Can you work these out from the model? Positions are in its coordinate system, mm. Face numbers are marked on the shaded views. A direction names the side the tool comes from. Coordinates: 2 decimals unless noted, no trailing zeros. Loops run counter-clockwise (first coordinate to the right, second up) from the corner with the lowest first, then second, coordinate; pieces in that order, holes last.
```python
from build123d import *
from OCP.BRepFilletAPI import BRepFilletAPI_MakeChamfer

# Parameters (mm, degrees)
SKETCH1_W                    = 2.54
SKETCH1_H                    = 2.54
BOSS_EXTRUDE1_DEPTH          = 2.54
BOSS_EXTRUDE2_START          = -5.64
SKETCH2_W                    = 0.65
SKETCH2_H                    = 0.65
BOSS_EXTRUDE2_DEPTH          = 11.34
CHAMFER1_SIZE                = 0.3
CHAMFER1_SIZE2               = 0.091719204
CHAMFER3_SIZE                = 0.7
CHAMFER3_SIZE2               = 0.341412812
CHAMFER4_SIZE                = 0.7
CHAMFER4_SIZE2               = 0.341412812
R_P_TITION_START             = -1.27
R_P_TITION_LIN_AIRE3_DEPTH   = 2.54
R_P_TITION_START_2           = -0.325
R_P_TITION_LIN_AIRE3_2_DEPTH = 0.65
R_P_TITION_START_3           = 1.611412812
R_P_TITION_LIN_AIRE3_3_DEPTH = 4.397174376
R_P_TITION_START_4           = -1
R_P_TITION_LIN_AIRE3_4_DEPTH = 5


with BuildPart() as part:
    # Sketch1 → Boss-Extrude1 (new body)
    with BuildSketch(Plane(origin=(0, 0, 0), x_dir=(1, 0, 0), z_dir=(0, 1, 0))):
        Rectangle(SKETCH1_W, SKETCH1_H)
    extrude(amount=BOSS_EXTRUDE1_DEPTH)

    # Sketch2 → Boss-Extrude2 (add)
    with BuildSketch(Plane(origin=(0, 2.54, 0), x_dir=(1, 0, 0), z_dir=(0, 1, 0)).offset(BOSS_EXTRUDE2_START)):
        Rectangle(SKETCH2_W, SKETCH2_H)
    extrude(amount=BOSS_EXTRUDE2_DEPTH)

    # Chamfer1: one chamfer whose edges measure the first distance from different faces: ONE call of the kernel's chamfer builder (chamfer() names one face for all edges)
    chamfer1_edges_1 = [part.edges().sort_by_distance(p)[0] for p in [
        (-0.325, -3.1, 0),
        (0, -3.1, -0.325),
        (0.325, -3.1, 0),
        (0, -3.1, 0.325),
    ]]
    chamfer1_side_1 = [part.faces().sort_by_distance(p)[0] for p in [
        (0, -3.1, 0),
    ]]
    chamfer1_edges_2 = [part.edges().sort_by_distance(p)[0] for p in [
        (-0.325, 8.24, 0),
    ]]
    chamfer1_side_2 = [part.faces().sort_by_distance(p)[0] for p in [
        (-0.325, 5.39, 0),
    ]]
    chamfer1_edges_3 = [part.edges().sort_by_distance(p)[0] for p in [
        (0, 8.24, 0.325),
    ]]
    chamfer1_side_3 = [part.faces().sort_by_distance(p)[0] for p in [
        (0, 5.39, 0.325),
    ]]
    chamfer1_edges_4 = [part.edges().sort_by_distance(p)[0] for p in [
        (0.325, 8.24, 0),
    ]]
    chamfer1_side_4 = [part.faces().sort_by_distance(p)[0] for p in [
        (0.325, 5.39, 0),
    ]]
    chamfer1_edges_5 = [part.edges().sort_by_distance(p)[0] for p in [
        (0, 8.24, -0.325),
    ]]
    chamfer1_side_5 = [part.faces().sort_by_distance(p)[0] for p in [
        (0, 5.39, -0.325),
    ]]
    chamfer1 = BRepFilletAPI_MakeChamfer(part.part.solid().wrapped)
    for e in chamfer1_edges_1:
        chamfer1.Add(CHAMFER1_SIZE, CHAMFER1_SIZE2, e.wrapped, chamfer1_side_1[0].wrapped)  # the first distance lies on this face
    for e in chamfer1_edges_2:
        chamfer1.Add(CHAMFER1_SIZE, CHAMFER1_SIZE2, e.wrapped, chamfer1_side_2[0].wrapped)  # the first distance lies on this face
    for e in chamfer1_edges_3:
        chamfer1.Add(CHAMFER1_SIZE, CHAMFER1_SIZE2, e.wrapped, chamfer1_side_3[0].wrapped)  # the first distance lies on this face
    for e in chamfer1_edges_4:
        chamfer1.Add(CHAMFER1_SIZE, CHAMFER1_SIZE2, e.wrapped, chamfer1_side_4[0].wrapped)  # the first distance lies on this face
    for e in chamfer1_edges_5:
        chamfer1.Add(CHAMFER1_SIZE, CHAMFER1_SIZE2, e.wrapped, chamfer1_side_5[0].wrapped)  # the first distance lies on this face
    add(Compound.cast(chamfer1.Shape()), mode=Mode.REPLACE)

    # Chamfer3
    chamfer3_edges = [part.edges().sort_by_distance(p)[0] for p in [
        (1.27, 2.54, 0),
        (1.27, 1.27, 1.27),
        (1.27, 1.27, -1.27),
    ]]
    chamfer3_side = [part.faces().sort_by_distance(p)[0] for p in [
        (1.27, 1.27, 0),
    ]]
    chamfer(chamfer3_edges, length=CHAMFER3_SIZE, length2=CHAMFER3_SIZE2, reference=chamfer3_side[0])

    # Chamfer4
    chamfer4_edges = [part.edges().sort_by_distance(p)[0] for p in [
        (-1.27, 2.54, 0),
        (-1.27, 1.27, 1.27),
        (-1.27, 1.27, -1.27),
    ]]
    chamfer4_side = [part.faces().sort_by_distance(p)[0] for p in [
        (-1.27, 1.27, 0),
    ]]
    chamfer(chamfer4_edges, length=CHAMFER4_SIZE, length2=CHAMFER4_SIZE2, reference=chamfer4_side[0])

    # Répétition linéaire3: read off the stored shape, not the designer's step
    # Répétition linéaire3 outline → Répétition linéaire3 (add)
    with BuildSketch(Plane.XY.offset(R_P_TITION_START)):
        Polygon((3.468587188, 2.54), (1.611412812, 2.54), (1.27, 1.84), (1.27, 0), (6.35, 0), (6.35, 1.84), (6.008587188, 2.54), (4.151412812, 2.54), (3.81, 1.84), align=None)
    extrude(amount=R_P_TITION_LIN_AIRE3_DEPTH)

    # R_p_tition lin_aire3 2 outline → R_p_tition lin_aire3 2 (add)
    with BuildSketch(Plane.XY.offset(R_P_TITION_START_2)):
        Polygon((2.215, 7.94), (2.215, 2.54), (2.865, 2.54), (2.865, 7.94), (2.773280796, 8.24), (2.306719204, 8.24), align=None)
        Polygon((2.865, 0), (2.215, 0), (2.215, -3.008280796), (2.515, -3.1), (2.565, -3.1), (2.865, -3.008280796), align=None)
        Polygon((5.405, 0), (4.755, 0), (4.755, -3.008280796), (5.055, -3.1), (5.105, -3.1), (5.405, -3.008280796), align=None)
        Polygon((4.755, 7.94), (4.755, 2.54), (5.405, 2.54), (5.405, 7.94), (5.313280796, 8.24), (4.846719204, 8.24), align=None)
    extrude(amount=R_P_TITION_LIN_AIRE3_2_DEPTH)

    # R_p_tition lin_aire3 3 outline → R_p_tition lin_aire3 3 (cut)
    with BuildSketch(Plane.YZ.offset(R_P_TITION_START_3)):
        Polygon((-3.1, 0.025), (-3.008280796, 0.325), (-3.1, 0.325), align=None)
        Polygon((-3.008280796, -0.325), (-3.1, -0.025), (-3.1, -0.325), align=None)
        Polygon((8.24, 0.325), (7.94, 0.325), (8.24, 0.233280796), align=None)
        Polygon((8.24, -0.325), (8.24, -0.233280796), (7.94, -0.325), align=None)
    extrude(amount=R_P_TITION_LIN_AIRE3_3_DEPTH, mode=Mode.SUBTRACT)

    # R_p_tition lin_aire3 4 outline → R_p_tition lin_aire3 4 (cut)
    with BuildSketch(Plane(origin=(0, 0, 0), x_dir=(1, 0, 0), z_dir=(0, 1, 0)).offset(R_P_TITION_START_4)):
        Polygon((4.151412812, -1.27), (3.81, -0.57), (3.468587188, -1.27), align=None)
        Polygon((1.27, 0.57), (1.611412812, 1.27), (1.27, 1.27), align=None)
        Polygon((3.81, 0.57), (4.151412812, 1.27), (3.468587188, 1.27), align=None)
        Polygon((6.008587188, 1.27), (6.35, 0.57), (6.35, 1.27), align=None)
        Polygon((6.35, -0.57), (6.008587188, -1.27), (6.35, -1.27), align=None)
        Polygon((1.27, -1.27), (1.611412812, -1.27), (1.27, -0.57), align=None)
    extrude(amount=R_P_TITION_LIN_AIRE3_4_DEPTH, mode=Mode.SUBTRACT)


solid = part.part
```
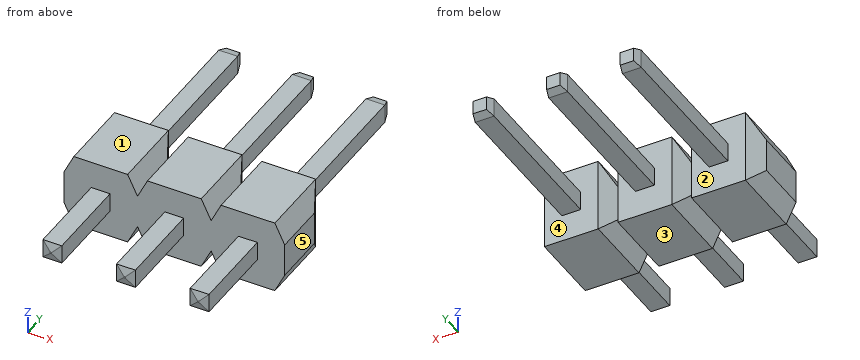
(1) If we mould it in two halves opening along X, with no side actions, what happens to the marked faces 3, 4 and 5? For each: released by +X, released by -X, zero draft, split by the parting line, or undercut.
Check values:
face 3: zero draft
face 4: undercut
face 5: released by +X
(2) Which directions (+Z, -Z, +X, -X, +Y, -Y) give clear straight access to the entire face, cutting with the end or side of a thin tool? Please do the marked faces 1 and 2.
Check values:
face 1: +Z, +X, -X, +Y, -Y
face 2: +Y
(3) I'm going to push flat-ended pins straight in: pin 1 (1.5 mm diameter, centred on y = 5.5, z = -1, fed in from -X) (3 decimals); pin 2 (0.5 mm diameter, centred on x = 2.5, y = 4, fed in from -Z) (3 decimals); pin 3 (0.5 mm diameter, centred on x = 2.5, y = 5, fed in from +Z) (3 decimals). Where does each tip first touch, or does it pass through?
Check values:
pin 1: stops at x = -0.325
pin 2: stops at z = -0.325
pin 3: stops at z = 0.325
(4) I want a section at B-B on z = -0.8. Write out the boundary of the cut face in (x, y).
Check values:
outline: (-1.16, 0) - (1.16, 0) - (1.16, 2.07) - (0.93, 2.54) - (-0.93, 2.54) - (-1.16, 2.07) - close; (1.38, 0) - (3.7, 0) - (3.7, 2.07) - (3.47, 2.54) - (1.61, 2.54) - (1.38, 2.07) - close; (3.92, 0) - (6.24, 0) - (6.24, 2.07) - (6.01, 2.54) - (4.15, 2.54) - (3.92, 2.07) - close
(5) I want a section at A-A on y = 0.75. Write out the boundary of the cut face in (x, z).
Check values:
outline: (-1.27, -0.57) - (-0.93, -1.27) - (0.93, -1.27) - (1.27, -0.57) - (1.61, -1.27) - (3.47, -1.27) - (3.81, -0.57) - (4.15, -1.27) - (6.01, -1.27) - (6.35, -0.57) - (6.35, 0.57) - (6.01, 1.27) - (4.15, 1.27) - (3.81, 0.57) - (3.47, 1.27) - (1.61, 1.27) - (1.27, 0.57) - (0.93, 1.27) - (-0.93, 1.27) - (-1.27, 0.57) - close
(6) I want a section at C-C on y = 2.75. Write out the boundary of the cut face in (x, z) (3 decimals).
Check values:
outline: (-0.325, -0.325) - (0.325, -0.325) - (0.325, 0.325) - (-0.325, 0.325) - close; (2.215, -0.325) - (2.865, -0.325) - (2.865, 0.325) - (2.215, 0.325) - close; (4.755, -0.325) - (5.405, -0.325) - (5.405, 0.325) - (4.755, 0.325) - close
(7) If I drill on probe 1 along X at (y, z) = (3.5, -0.25) (3 decimals); probe 2 along Y at (x, z) = (1.75, 0.6); probe 3 along Z at (x, y) = (2.75, 7.5) (3 decimals), over which ranges is the centre line in solid material (lowest first)?
Check values:
probe 1: x = -0.325 to 0.325, 2.215 to 2.865, 4.755 to 5.405
probe 2: y = 0 to 2.54
probe 3: z = -0.325 to 0.325
(8) I want a section at D-D on x = 4.5. Write out the boundary of the cut face in (y, z).
Check values:
outline: (0, -1.27) - (2.54, -1.27) - (2.54, 1.27) - (0, 1.27) - close
